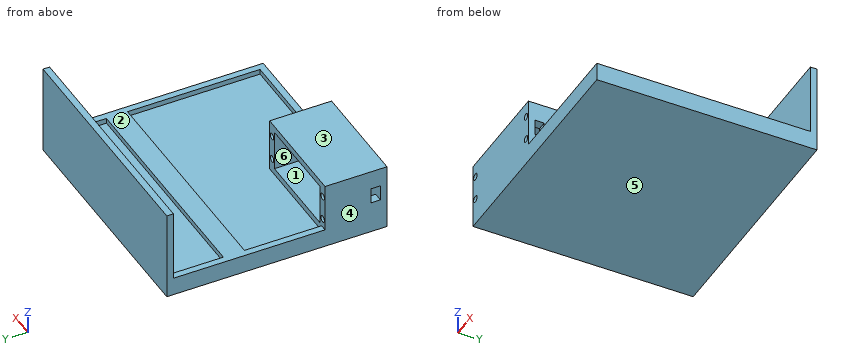
```python
from build123d import *

# Parameters (mm, degrees)
SKETCH2_W                = 81
SKETCH2_H                = 41
SKETCH2_W_2              = 67
SKETCH2_H_2              = 31
BOSS_EXTRUDE1_DEPTH      = 42
BOSS_EXTRUDE1_DEPTH_BACK = 5
BOSS_EXTRUDE2_REACH      = 76
SKETCH3_W                = 31
SKETCH3_H                = 5
SKETCH4_R                = 2.5
CUT_EXTRUDE1_DEPTH       = 48
SKETCH5_W                = 12
SKETCH5_H                = 7
CUT_EXTRUDE2_DEPTH       = 20
SKETCH6_W                = 81
SKETCH6_H                = 47
BOSS_EXTRUDE3_DEPTH      = 10
SKETCH7_W                = 81
SKETCH7_H                = 10
BOSS_EXTRUDE4_DEPTH      = 120
SKETCH9_W                = 10
SKETCH9_H                = 167
BOSS_EXTRUDE6_DEPTH      = 100
SKETCH8_W                = 181
SKETCH8_H                = 16
BOSS_EXTRUDE5_DEPTH      = 4
SKETCH11_W               = 95
SKETCH11_H               = 5
SKETCH11_W_2             = 5
SKETCH11_H_2             = 100.5
SKETCH11_H_3             = 45.5
SKETCH11_W_3             = 181
SKETCH11_H_4             = 58.5
BOSS_EXTRUDE7_DEPTH      = 4
SKETCH12_W               = 181
SKETCH12_H               = 5
BOSS_EXTRUDE8_DEPTH      = 55


with BuildPart() as part:
    # Sketch2 → Boss-Extrude1 (new body, two sides)
    with BuildSketch(Plane(origin=(0, 0, 0), x_dir=(1, 0, 0), z_dir=(0, 1, 0))) as boss_extrude1_sk:
        Rectangle(SKETCH2_W, SKETCH2_H)
        Rectangle(SKETCH2_W_2, SKETCH2_H_2, mode=Mode.SUBTRACT)
    extrude(amount=BOSS_EXTRUDE1_DEPTH)
    extrude(boss_extrude1_sk.sketch, amount=-BOSS_EXTRUDE1_DEPTH_BACK)

    # Sketch3 → Boss-Extrude2 (add, up to next)
    with BuildSketch(Plane(origin=(-33.5, 0, 0), x_dir=(0, 0, -1), z_dir=(1, 0, 0)), mode=Mode.PRIVATE) as boss_extrude2_sk1:
        with Locations((0, -2.5)):
            Rectangle(SKETCH3_W, SKETCH3_H)
    boss_extrude2_tool1 = extrude(boss_extrude2_sk1.sketch, amount=BOSS_EXTRUDE2_REACH, mode=Mode.PRIVATE) - part.part
    add(boss_extrude2_tool1.solids().sort_by_distance((-33.5, -2.5, 0))[0])

    # Sketch4 → Cut-Extrude1 (cut, through all)
    with BuildSketch(Plane(origin=(0, 42, 0), x_dir=(1, 0, 0), z_dir=(0, 1, 0))):
        with Locations((-37, 9.5)):
            Circle(SKETCH4_R)
        with Locations((-37, -9.5)):
            Circle(SKETCH4_R)
    cut_extrude1 = extrude(amount=-CUT_EXTRUDE1_DEPTH, mode=Mode.SUBTRACT)

    # Sketch5 → Cut-Extrude2 (cut)
    with BuildSketch(Plane.ZY.offset(40.5)):
        with Locations((0, 3.5)):
            Rectangle(SKETCH5_W, SKETCH5_H)
    cut_extrude2 = extrude(amount=-CUT_EXTRUDE2_DEPTH, mode=Mode.SUBTRACT)

    # Mirror1: Cut-Extrude1, Cut-Extrude2 across plane
    add(cut_extrude1.mirror(Plane(origin=(0, 0, 0), x_dir=(0, 0, 1), z_dir=(1, 0, 0))), mode=Mode.SUBTRACT)
    add(cut_extrude2.mirror(Plane(origin=(0, 0, 0), x_dir=(0, 0, 1), z_dir=(1, 0, 0))), mode=Mode.SUBTRACT)

    # Sketch6 → Boss-Extrude3 (add)
    with BuildSketch(Plane(origin=(0, 0, -20.5), x_dir=(-1, 0, 0), z_dir=(0, 0, -1))):
        with Locations((0, 18.5)):
            Rectangle(SKETCH6_W, SKETCH6_H)
    extrude(amount=BOSS_EXTRUDE3_DEPTH)

    # Sketch7 → Boss-Extrude4 (add)
    with BuildSketch(Plane(origin=(0, 42, 0), x_dir=(1, 0, 0), z_dir=(0, 1, 0))):
        with Locations((0, 25.5)):
            Rectangle(SKETCH7_W, SKETCH7_H)
    extrude(amount=BOSS_EXTRUDE4_DEPTH)

    # Sketch9 → Boss-Extrude6 (add)
    with BuildSketch(Plane(origin=(40.5, 0, 0), x_dir=(0, 0, -1), z_dir=(1, 0, 0))):
        with Locations((25.5, 78.5)):
            Rectangle(SKETCH9_W, SKETCH9_H)
    extrude(amount=BOSS_EXTRUDE6_DEPTH)

    # Sketch8 → Boss-Extrude5 (add)
    with BuildSketch(Plane.XY.offset(-20.5)):
        with Locations((50, 108.5)):
            Rectangle(SKETCH8_W, SKETCH8_H)
    extrude(amount=BOSS_EXTRUDE5_DEPTH)

    # Sketch11 → Boss-Extrude7 (add)
    with BuildSketch(Plane.XY.offset(-20.5)):
        with Locations((88, -2.5)):
            Rectangle(SKETCH11_W, SKETCH11_H)
        with Locations((138, 50.25)):
            Rectangle(SKETCH11_W_2, SKETCH11_H_2)
        with Locations((138, -2.5)):
            Rectangle(SKETCH11_W_2, SKETCH11_H)
        with Locations((-38, 139.25)):
            Rectangle(SKETCH11_W_2, SKETCH11_H_3)
        with Locations((50, 159.5)):
            Rectangle(SKETCH11_W_3, SKETCH11_H)
        with Locations((138, 139.25)):
            Rectangle(SKETCH11_W_2, SKETCH11_H_3)
        with Locations((-38, 71.25)):
            Rectangle(SKETCH11_W_2, SKETCH11_H_4)
    extrude(amount=BOSS_EXTRUDE7_DEPTH)

    # Sketch12 → Boss-Extrude8 (add)
    with BuildSketch(Plane.XY.offset(-16.5)):
        with Locations((50, 159.5)):
            Rectangle(SKETCH12_W, SKETCH12_H)
    extrude(amount=BOSS_EXTRUDE8_DEPTH)


solid = part.part
```
Read the model definition and answer for the solid it produces. Units are mm, in the model's axes. Face numbers are marked on the shaded views. A direction names the side the tool comes from. Give positions to 0.01 mm unless a question says otherwise; leave off trailing zeros. Loops run counter-clockwise (first coordinate to the right, second up) from the corner with the lowest first, then second, coordinate; pieces in that order, holes last.
Item 1: The mould has two halves that part along X. Classify the marked faces 4, 5 and 6: released by +X, released by -X, zero draft, split by the parting line, or undercut.
Item 2: The part is cut by section B-B (z = -9.5). Write down the section's boundary in (x, y), and give its area (3 significant figures).
Item 3: For the marked faces 1, 2 and 3, determine the directions among +Z, -Z, +X, -X, +Y, -Y from which every point of the face is accessible in a straight line to the end or side of a thin tool.
Item 4: The part is cut by section D-D (y = 29). Write down the section's boundary in (x, z).
Item 5: Find the intervals of material crossed by line 1 along Z through (x, y) = (-37, 27); line 2 along X through (y, z) = (13, 9); line 3 along Y through (x, z) = (18, 18.5), in increasing order.
Item 6: The part is cut by section C-C (y = 132.5). Write down the section's boundary in (x, z), and give its area (3 significant figures).
Item 7: The part is cut by section A-A (x = 37). Write down the section's boundary in (y, z).
Item 8: Each of these flat-tipped pins is pushed along its axis until it touches: pin 1 Ø5 at (x, y) = (35, 64.5) entering from +Z; pin 2 Ø5 at (x, z) = (52.5, -10.5) entering from -Y; pin 3 Ø2 at (x, y) = (-37.5, 5) entering from +Z. Where does it stop, or does it pass through?
Taken from the geometry:
1. face 4: released by -X
1. face 5: zero draft
1. face 6: undercut
2. outline: (-40.5, -5) - (-39.5, -5) - (-39.5, 42) - (-40.5, 42) - close; (-40.5, 157) - (140.5, 157) - (140.5, 162) - (-40.5, 162) - close; (-34.5, -5) - (34.5, -5) - (34.5, 42) - (33.5, 42) - (33.5, 0) - (-33.5, 0) - (-33.5, 42) - (-34.5, 42) - close; (39.5, -5) - (40.5, -5) - (40.5, 42) - (39.5, 42) - close
2. area: 1,430 mm2
3. face 1: none
3. face 2: +Z, +X
3. face 3: +Z, +X, -X, -Y
4. outline: (-40.5, -30.5) - (140.5, -30.5) - (140.5, -16.5) - (135.5, -16.5) - (135.5, -20.5) - (40.5, -20.5) - (40.5, 20.5) - (-40.5, 20.5) - close; hole circle Ø5 at (-37, -9.5); hole circle Ø5 at (-37, 9.5); hole (-33.5, -15.5) - (33.5, -15.5) - (33.5, 15.5) - (-33.5, 15.5) - close; hole circle Ø5 at (37, -9.5); hole circle Ø5 at (37, 9.5)
5. line 1: z = -30.5 to -12, -7 to 7, 12 to 20.5
5. line 2: x = -40.5 to -39.45, -34.55 to -33.5, 33.5 to 34.55, 39.45 to 40.5
5. line 3: y = -5 to 42, 157 to 162
6. outline: (-40.5, -30.5) - (140.5, -30.5) - (140.5, -16.5) - (135.5, -16.5) - (135.5, -20.5) - (-35.5, -20.5) - (-35.5, -16.5) - (-40.5, -16.5) - close
6. area: 1,850 mm2
7. outline: (-5, -30.5) - (162, -30.5) - (162, 38.5) - (157, 38.5) - (157, -20.5) - (116.5, -20.5) - (116.5, -16.5) - (100.5, -16.5) - (100.5, -20.5) - (42, -20.5) - (42, -12) - (-5, -12) - close; (-5, -7) - (42, -7) - (42, 7) - (-5, 7) - close; (-5, 12) - (42, 12) - (42, 20.5) - (-5, 20.5) - close; hole (0, -6) - (7, -6) - (7, 6) - (0, 6) - close
8. pin 1: stops at z = -20.5
8. pin 2: stops at y = 157
8. pin 3: stops at z = 20.5
